Drawing for the job (mm, zero at the part's lowest x, y, z). Coordinates: 2 decimals unless noted, no trailing zeros. Write each loop counter-clockwise with the first axis right and the second up, starting at its lowest first coordinate (ties: lowest second). Pieces come first, ordered by that corner, then holes. Notation, with made-up numbers: M -8.75,-38 L 7.25,-38 A36 cw 7.25,-4 Z; hole C 53.25,-16.5 d7. An arc over 180 degrees is marked long. Use CSV: the item, a comma, the result in double quotes. Start each with the question number.
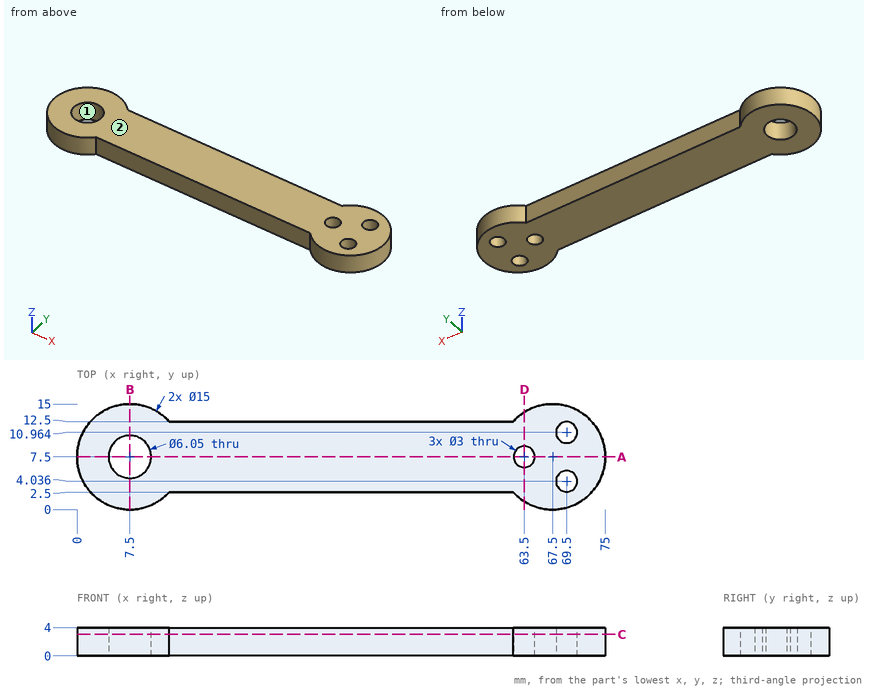
1) Band-saw the part on B-B on x = 7.5. List the corners of the cut face in (y, z) (3 decimals).
2) Two-plate mould, pull along X, no slides. Class the marked faces 1 and 2: pulls with the +X half, pulls with the -X half, needs draft (parallel to the pull), parting line crosses it, or undercut.
3) Band-saw the part on C-C on z = 3.05. List the corners of the cut face in (x, y) (3 decimals).
4) Drop flat-ended pins along their axis: P1, Ø2, axis at y = 11, z = 3, coming from the +X side; P2, Ø1.2, axis at x = 39.5, z = 1, coming from the +Y side; P3, Ø2, axis at x = 42.5, z = 2, coming from the -Y side. Give the stop position or say it passes through.
5) Wall check: L1, parallel to X at y = 5.25, z = 3.1 (1 decimal); L2, parallel to Y at x = 7.5, z = 2.75 (3 decimals); L3, parallel to X at y = 8.5, z = 0.5 (1 decimal). Give the ranges that are in metal, low to high. Write a range as [from, to].
6) Band-saw the part on D-D on x = 63.5. List the corners of the cut face in (y, z).
7) Band-saw the part on A-A on y = 7.5. List the corners of the cut face in (x, z) (3 decimals), then the cut area to 3 significant figures.
Findings below:
1,outline,"M 0,0 L 4.475,0 L 4.475,4 L 0,4 Z; M 10.525,0 L 15,0 L 15,4 L 10.525,4 Z"
2,face 1,"undercut"
2,face 2,"needs draft"
3,outline,"M 13.09,2.5 L 61.91,2.5 A7.5 ccw long 61.91,12.5 L 13.09,12.5 A7.5 ccw long Z; hole C 7.5,7.5 d6.05; hole C 63.5,7.5 d3; hole C 69.5,4.036 d3; hole C 69.5,10.964 d3"
4,P1,"stops at x = 74.57"
4,P2,"stops at y = 12.5"
4,P3,"stops at y = 2.5"
5,L1,"x = [0.3, 5.5], [9.5, 68.6], [70.4, 74.7]"
5,L2,"y = [0, 4.475], [10.525, 15]"
5,L3,"x = [0.1, 4.6], [10.4, 62.4], [64.6, 74.9]"
6,outline,"M 1.16,0 L 6,0 L 6,4 L 1.16,4 Z; M 9,0 L 13.84,0 L 13.84,4 L 9,4 Z"
7,outline,"M 0,0 L 4.475,0 L 4.475,4 L 0,4 Z; M 10.525,0 L 62,0 L 62,4 L 10.525,4 Z; M 65,0 L 75,0 L 75,4 L 65,4 Z"
7,area,"264 mm2"
